The figure shows three views and two pictorial views of one solid part (mm, origin at its lowest corner). Answer the questions. Coordinates: 2 decimals unless noted, no trailing zeros. Write each loop counter-clockwise with the first axis right and the second up, starting at its lowest first coordinate (ties: lowest second). Pieces come first, ordered by that corner, then holes.
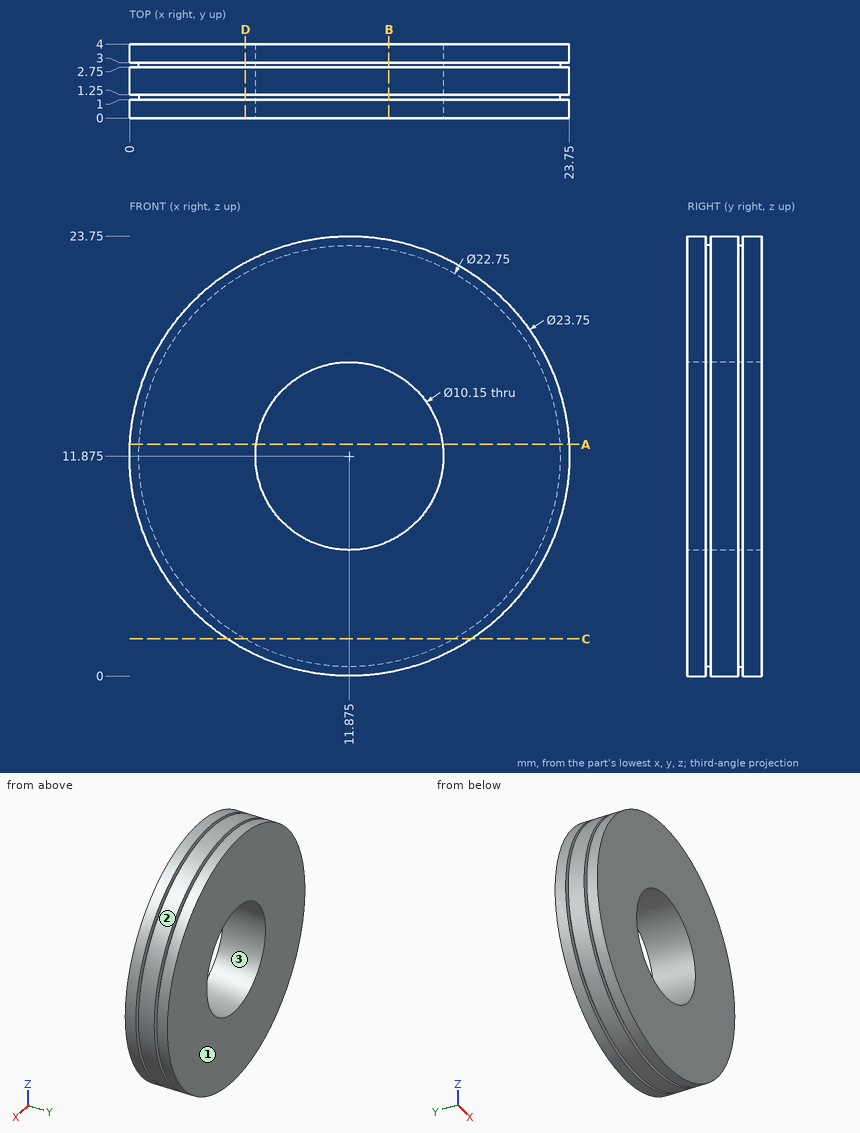
Q1. Given pin 1 (2 mm diameter, centred on x = 6.5, z = 5.5, fed in from -Y); pin 2 (2 mm diameter, centred on x = 18, y = 3.5, fed in from -Z), each flat-ended and moving along its own axis, determine where each tip first touches the part or whether it passes through.
Answers below:
pin 1: stops at y = 0
pin 2: stops at z = 1.16
Q2. Determine the mould class of the marked faces 1, 2 and 3 for opening direction X: released by +X, released by -X, zero draft, split by the parting line, or undercut.
Answers below:
face 1: zero draft
face 2: split by the parting line
face 3: undercut
Q3. The part is cut by section A-A, the plane z = 12.5. Write down the section's boundary in (x, y), then the cut area to 3 significant figures.
Answers below:
outline: (0.02, 0) - (6.84, 0) - (6.84, 4) - (0.02, 4) - (0.02, 3) - (0.52, 3) - (0.52, 2.75) - (0.02, 2.75) - (0.02, 1.25) - (0.52, 1.25) - (0.52, 1) - (0.02, 1) - close; (16.91, 0) - (23.73, 0) - (23.73, 1) - (23.23, 1) - (23.23, 1.25) - (23.73, 1.25) - (23.73, 2.75) - (23.23, 2.75) - (23.23, 3) - (23.73, 3) - (23.73, 4) - (16.91, 4) - close
area: 54.1 mm2
Q4. The part is cut by section C-C, the plane z = 2. Write down the section's boundary in (x, y), then the cut area to 3 significant figures.
Answers below:
outline: (5.28, 0) - (18.47, 0) - (18.47, 1) - (17.52, 1) - (17.52, 1.25) - (18.47, 1.25) - (18.47, 2.75) - (17.52, 2.75) - (17.52, 3) - (18.47, 3) - (18.47, 4) - (5.28, 4) - (5.28, 3) - (6.23, 3) - (6.23, 2.75) - (5.28, 2.75) - (5.28, 1.25) - (6.23, 1.25) - (6.23, 1) - (5.28, 1) - close
area: 51.8 mm2
Q5. The part is cut by section D-D, the plane x = 6.25. Write down the section's boundary in (y, z), then the cut area to 3 significant figures.
Answers below:
outline: (0, 1.42) - (1, 1.42) - (1, 1.99) - (1.25, 1.99) - (1.25, 1.42) - (2.75, 1.42) - (2.75, 1.99) - (3, 1.99) - (3, 1.42) - (4, 1.42) - (4, 22.33) - (3, 22.33) - (3, 21.76) - (2.75, 21.76) - (2.75, 22.33) - (1.25, 22.33) - (1.25, 21.76) - (1, 21.76) - (1, 22.33) - (0, 22.33) - close
area: 83.1 mm2
Q6. Find the intervals of material crossed by probe 1 along X at (y, z) = (3.55, 12); probe 2 along Z at (x, y) = (12.5, 1.2); probe 3 along Z at (x, y) = (16.5, 0.85), in increasing order.
Answers below:
probe 1: x = 0 to 6.8, 16.95 to 23.75
probe 2: z = 0.52 to 6.84, 16.91 to 23.23
probe 3: z = 0.94 to 9.79, 13.96 to 22.81
Q7. The part is cut by section B-B, the plane x = 14. Write down the section's boundary in (y, z).
Answers below:
outline: (0, 0.19) - (1, 0.19) - (1, 0.7) - (1.25, 0.7) - (1.25, 0.19) - (2.75, 0.19) - (2.75, 0.7) - (3, 0.7) - (3, 0.19) - (4, 0.19) - (4, 7.27) - (0, 7.27) - close; (0, 16.48) - (4, 16.48) - (4, 23.56) - (3, 23.56) - (3, 23.05) - (2.75, 23.05) - (2.75, 23.56) - (1.25, 23.56) - (1.25, 23.05) - (1, 23.05) - (1, 23.56) - (0, 23.56) - close
